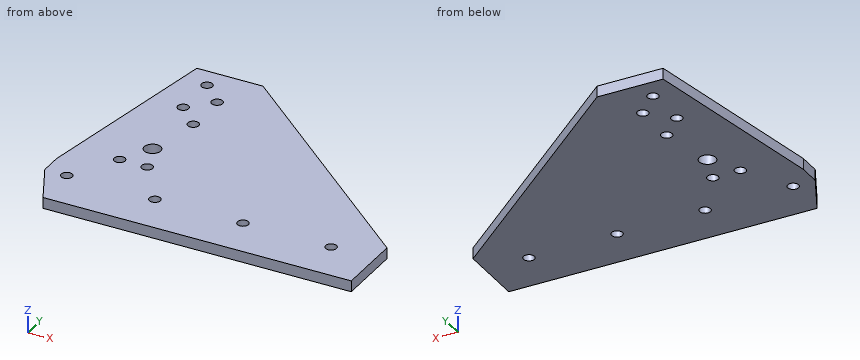
Autodesk Inventor part; units mm, degrees
ref_plane "YZ Plane" through (0, 0, 0) normal (1, 0, 0) x (0, 1, 0)
ref_plane "XZ Plane" through (0, 0, 0) normal (0, 1, 0) x (-1, 0, 0)
ref_plane "XY Plane" through (0, 0, 0) normal (0, 0, 1) x (1, 0, 0)
sketch "Sketch1" plane through (0, 0, 0) normal (0, 0, 1) x (1, 0, 0)
  line L0 (0, 0) -> (190.5, 0) construction
  line L1 (190.5, 0) -> (190.5, 152.4) construction
  line L2 (190.5, 152.4) -> (0, 152.4) construction
  line L3 (0, 152.4) -> (0, 0) construction
  line L4 (0, 0) -> (190.5, 0)
  line L5 (0, 0) -> (0, 38.1)
  line L6 (0, 0) -> (38.1, 0) construction
  line L7 (190.5, 0) -> (190.5, 38.1)
  line L8 (190.5, 0) -> (228.6, 0) construction
  line L9 (190.5, 152.4) -> (57.15, 152.4) construction
  line L10 (190.5, 152.4) -> (323.85, 152.4) construction
  line L11 (57.15, 152.4) -> (19.05, 152.4) construction
  line L12 (0, 38.1) -> (19.05, 152.4)
  line L13 (19.05, 152.4) -> (57.15, 152.4)
  line L14 (57.15, 152.4) -> (190.5, 38.1)
  circle A0 centre (12.7, 25.4) radius 3.175
  circle A1 centre (63.5, 25.4) radius 3.175
  circle A2 centre (31.75, 139.7) radius 3.175
  circle A3 centre (44.45, 127) radius 3.175
  circle A4 centre (31.75, 114.3) radius 3.175
  circle A5 centre (44.45, 101.6) radius 3.175
  circle A6 centre (114.3, 25.4) radius 3.175
  circle A7 centre (165.1, 25.4) radius 3.175
  dimension "d0" = 190.5
  dimension "d1" = 152.4
  dimension "d2" = 12.7
  dimension "d3" = 50.8
  dimension "d8" = 25.4
  dimension "d9" = 25.4
  dimension "d10" = 38.1
  dimension "d11" = 90
  dimension "d12" = 38.1
  dimension "d13" = 90
  dimension "d14" = 133.35
  dimension "d15" = 180
  dimension "d16" = 38.1
  dimension "d17" = 12.7
  dimension "d18" = 12.7
  dimension "d19" = 12.7
  dimension "d20" = 12.7
  dimension "d21" = 12.7
  dimension "d22" = 25.4
  dimension "d23" = 38.1
  dimension "d24" = 50.8
  dimension "d25" = 6.35
  dimension "d26" = 6.35
  dimension "d29" = 6.35
  dimension "d30" = 6.35
  dimension "d31" = 6.35
  dimension "d32" = 6.35
  dimension "d35" = 50.8
  dimension "d36" = 50.8
  dimension "d38" = 6.35
  dimension "d39" = 6.35
  dimension "d46" = 25.4
  dimension "d47" = 25.4
extrude "Extrusion4" add sketch "Sketch1" along normal blind 6.35
sketch "Sketch3" plane through (0, 0, 6.35) normal (0, 0, 1) x (1, 0, 0)
  line L0 (0, 0) -> (0, 25.4)
  line L1 (0, 38.1) -> (0, 0)
  line L2 (0, 0) -> (12.7, 0)
  line L3 (0, 0) -> (190.5, 0)
  line L4 (0, 25.4) -> (12.7, 0)
  dimension "d50" = 25.4
  dimension "d51" = 12.7
extrude "Extrusion5" cut sketch "Sketch3" against normal blind 6.35
sketch "Sketch4" plane through (0, 0, 6.35) normal (0, 0, 1) x (1, 0, 0)
  line L0 (0, 38.1) -> (0, 25.4)
  line L1 (12.7, 0) -> (190.5, 0)
  circle A0 centre (28.575, 52.3875) radius 3.175
  circle A1 centre (44.45, 52.3875) radius 3.175
  circle A2 centre (38.1, 69.85) radius 4.7625
  point P0 (0, 0)
  dimension "d54" = 28.575
  dimension "d55" = 44.45
  dimension "d56" = 52.3875
  dimension "d57" = 52.3875
  dimension "d58" = 69.85
  dimension "d59" = 38.1
  dimension "d60" = 6.35
  dimension "d61" = 6.35
  dimension "d62" = 9.525
extrude "Extrusion6" cut sketch "Sketch4" against normal blind 6.35
properties part number "rail mounting bracket"
Can you work these out from the model? Positions are in its coordinate system, mm. Give positions to 0.01 mm unless a question says otherwise; leave off trailing zeros. Loops run counter-clockwise (first coordinate to the right, second up) from the corner with the lowest first, then second, coordinate; pieces in that order, holes last. Notation, with made-up numbers: (69, 4.25) -> (100, 4.25) arc R18 cw to (100, 34.25) -> close; hole circle Ø8 at (33.5, 82.5). An arc over 180 degrees is marked (long way). Return JSON: item names as keys, results as strings.
Q1. I want a section at A-A, the plane y = 114.3. List the corners of the cut face in (x, z) for me (3 decimals), then the cut area to 3 significant figures.
Checks:
{"outline": "(12.7, 0) -> (28.575, 0) -> (28.575, 6.35) -> (12.7, 6.35) -> close; (34.925, 0) -> (101.6, 0) -> (101.6, 6.35) -> (34.925, 6.35) -> close", "area": "524 mm2"}
Q2. I want a section at B-B, the plane x = 63.5. List the corners of the cut face in (y, z) for me (3 decimals).
Checks:
{"outline": "(0, 0) -> (22.225, 0) -> (22.225, 6.35) -> (0, 6.35) -> close; (28.575, 0) -> (146.957, 0) -> (146.957, 6.35) -> (28.575, 6.35) -> close"}
Q3. I want a section at C-C, the plane z = 3.25. Count the separate pieces of the cut face and the enclosed holes in it, then the cut area to 3 significant figures.
Checks:
{"separate pieces": "1", "enclosed holes": "11", "area": "19,800 mm2"}
Q4. For pin 1 Ø15 at (x, y) = (38.1, 69.85) entering from +Z; pin 2 Ø3 at (x, z) = (140.5, 5) entering from +Y; pin 3 Ø1 at (y, z) = (42, 2) entering from +X, each with a flat end and sliding along its axis, tell me the tip position at first contact or that it passes through.
Checks:
{"pin 1": "stops at z = 6.35", "pin 2": "stops at y = 82.24", "pin 3": "stops at x = 186.53"}
Q5. I want a section at D-D, the plane x = 106.5. List the corners of the cut face in (y, z) for me, then the cut area to 3 significant figures.
Checks:
{"outline": "(0, 0) -> (110.1, 0) -> (110.1, 6.35) -> (0, 6.35) -> close", "area": "699 mm2"}
Q6. I need wall thicknesses on probe 1 along Y at (x, z) = (44.45, 2.25) (1 decimal); probe 2 along X at (y, z) = (25, 1.5); probe 3 along Y at (x, z) = (38.1, 3.25). Which ranges of each line are inside material? Lowest first, please.
Checks:
{"probe 1": "y = 0 to 49.2, 55.6 to 98.4, 104.8 to 123.8, 130.2 to 152.4", "probe 2": "x = 0.2 to 9.55, 15.85 to 60.35, 66.65 to 111.15, 117.45 to 161.95, 168.25 to 190.5", "probe 3": "y = 0 to 65.09, 74.61 to 152.4"}
